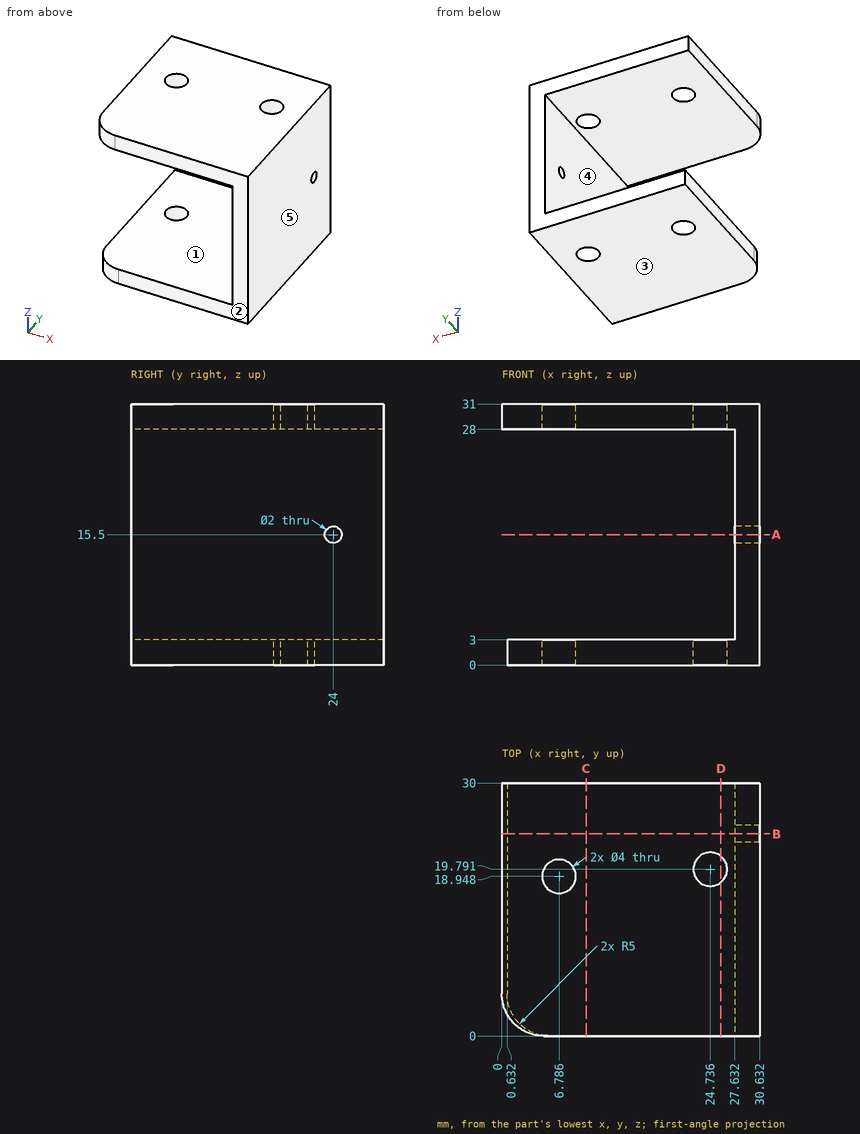
Could you check a few things on this drawing? It's one solid part, dimensions in mm from its lowest x, y, z. A direction names the side the tool comes from. Coordinates: 2 decimals unless noted, no trailing zeros. Order: outer loops, then holes, each group sorted by start corner. A loop starts at its lowest first (then second) coordinate and runs counter-clockwise, first axis right, second up. Notation, with made-up numbers: M 88.25,77 L 124.25,77 A9 cw 124.25,85 Z; hole C 58.5,1 d2. An arc over 180 degrees is marked long. Answer as a JSON object with one key per item and string values. Group by question number.
(1) Suppose I cut it at D-D, the plane x = 26. Please give me the cut outline in (y, z).
(2) Suppose I cut it at B-B, the plane y = 24. Please give me the cut outline in (x, z), then the cut area to 3 significant figures.
(3) Suppose I cut it at C-C, the plane x = 10. Please give me the cut outline in (y, z), then the cut area to 3 significant figures.
(4) Suppose I cut it at A-A, the plane z = 15.5. Please give me the cut outline in (x, y), then the cut area to 3 significant figures.
(5) If we mould it in two halves opening along Z, with no side actions, what happens to the marked faces 1, 2 and 3? For each: released by +Z, released by -Z, zero draft, split by the parting line, or undercut.
(6) Which directions (+Z, -Z, +X, -X, +Y, -Y) give clear straight access to the entire face, cutting with the end or side of a thin tool? Please do the marked faces 4 and 5.
(7) For pin 1 (3.5 mm diameter, centred on x = 24.74, y = 19.79, fed in from -Z); pin 2 (6 mm diameter, centred on y = 21, z = 23.5, fed in from -X); pin 3 (8 mm diameter, centred on x = 21.5, y = 11.5, fed in from -Z); pin 4 (0.9 mm diameter, centred on y = 20.5, z = 1.5, fed in from -X), each with a flat end and sliding along its axis, tell me the tip position at first contact or that it passes through.
(8) I need wall thicknesses on probe 1 along Z at (x, y) = (17.5, 26.25); probe 2 along Z at (x, y) = (2, 1.5); probe 3 along X at (y, z) = (12.5, 20). Which ranges of each line are inside material? Lowest first, please.
Values found:
{
 "1": {"outline": "M 0,0 L 18.24,0 L 18.24,3 L 0,3 Z; M 0,28 L 18.24,28 L 18.24,31 L 0,31 Z; M 21.34,0 L 30,0 L 30,3 L 21.34,3 Z; M 21.34,28 L 30,28 L 30,31 L 21.34,31 Z"},
 "2": {"outline": "M 0,28 L 27.63,28 L 27.63,16.5 L 30.63,16.5 L 30.63,31 L 0,31 Z; M 0.63,0 L 30.63,0 L 30.63,14.5 L 27.63,14.5 L 27.63,3 L 0.63,3 Z", "area": "251 mm^2"},
 "3": {"outline": "M 0,0 L 30,0 L 30,3 L 0,3 Z; M 0,28 L 30,28 L 30,31 L 0,31 Z", "area": "180 mm^2"},
 "4": {"outline": "M 27.63,0 L 30.63,0 L 30.63,23 L 27.63,23 Z; M 27.63,25 L 30.63,25 L 30.63,30 L 27.63,30 Z", "area": "84.0 mm^2"},
 "5": {"face 1": "undercut", "face 2": "zero draft", "face 3": "released by -Z"},
 "6": {"face 4": "-X, +Y, -Y", "face 5": "+Z, -Z, +X, +Y, -Y"},
 "7": {"pin 1": "passes through", "pin 2": "stops at x = 27.63", "pin 3": "stops at z = 0", "pin 4": "stops at x = 0.63"},
 "8": {"probe 1": "z = 0 to 3, 28 to 31", "probe 2": "z = 28 to 31", "probe 3": "x = 27.63 to 30.63"}
}
